```python
from build123d import *

# Parameters (mm, degrees)
SKETCH1_W           = 50.8
SKETCH1_H           = 50.8
SKETCH1_W_2         = 45.72
SKETCH1_H_2         = 45.72
BOSS_EXTRUDE1_DEPTH = 355.6
SKETCH2_R           = 14.2875
CUT_EXTRUDE1_DEPTH  = 50.8


with BuildPart() as part:
    # Sketch1 → Boss-Extrude1 (new body)
    with BuildSketch(Plane(origin=(0, 0, 0), x_dir=(1, 0, 0), z_dir=(0, 1, 0))):
        with Locations((25.4, -25.4)):
            Rectangle(SKETCH1_W, SKETCH1_H)
        with Locations((25.4, -25.4)):
            Rectangle(SKETCH1_W_2, SKETCH1_H_2, mode=Mode.SUBTRACT)
    extrude(amount=BOSS_EXTRUDE1_DEPTH)

    # Sketch2 → Cut-Extrude1 (cut)
    with BuildSketch(Plane.ZY):
        with Locations((25.4, 25.4)):
            Circle(SKETCH2_R)
    extrude(amount=-CUT_EXTRUDE1_DEPTH, mode=Mode.SUBTRACT)


solid = part.part
```
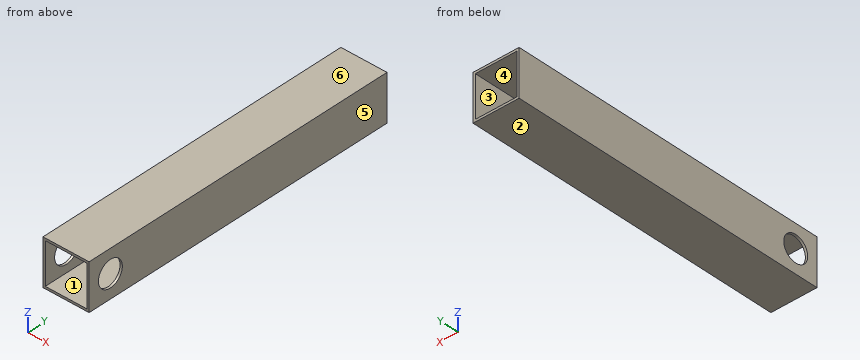
Verification items for the finished model (mm, model axes). Face numbers are marked on the shaded views. A direction names the side the tool comes from. Coordinates: 2 decimals unless noted, no trailing zeros. Write each loop counter-clockwise with the first axis right and the second up, starting at its lowest first coordinate (ties: lowest second). Pieces come first, ordered by that corner, then holes. Notation, with made-up numbers: M 22.25,-21 L 39.25,-21 A16 ccw 39.25,-15 Z; hole C 46,-20.75 d3. An arc over 180 degrees is marked long. Answer as a JSON object with one key per item and string values. Group by question number.
(1) Tool access check on the marked faces 1 and 2. Record the directions out of +Z, -Z, +X, -X, +Y, -Y that give a thin tool (end or side, any length) a straight path to the whole face; none if there is none.
(2) Material ranges on line 1 (X direction, y = 223, z = 12.5); line 2 (Y direction, x = 1.25, z = 25.4), recorded low to high.
(3) Cross-section at C-C, the plane y = 25.4. Record the cut outline in (x, z), and give its area (3 significant figures).
(4) Cross-section at A-A, the plane x = 24. Record the cut outline in (y, z), and give its area (3 significant figures).
(5) Cross-section at B-B, the plane z = 25.4. Record the cut outline in (x, y), and give its area (3 significant figures).
(6) Release check for a two-part mould opening along Z. For the marked faces 3, 4, 5 and 6 record: +Z half, -Z half, draft (parallel to the pull), parting line (faces both ways), or undercut.
(7) Cross-section at D-D, the plane z = 45. Record the cut outline in (x, y), and give its area (3 significant figures).
Reply:
{
 "1": {"face 1": "+Y, -Y", "face 2": "-Z, +X, -X, +Y, -Y"},
 "2": {"line 1": "0 to 2.54, 48.26 to 50.8", "line 2": "0 to 11.11, 39.69 to 355.6"},
 "3": {"outline": "M 0,0 L 50.8,0 L 50.8,11.11 L 48.26,11.11 L 48.26,2.54 L 2.54,2.54 L 2.54,11.11 L 0,11.11 Z; M 0,39.69 L 2.54,39.69 L 2.54,48.26 L 48.26,48.26 L 48.26,39.69 L 50.8,39.69 L 50.8,50.8 L 0,50.8 Z", "area": "345 mm²"},
 "4": {"outline": "M 0,0 L 355.6,0 L 355.6,2.54 L 0,2.54 Z; M 0,48.26 L 355.6,48.26 L 355.6,50.8 L 0,50.8 Z", "area": "1,810 mm²"},
 "5": {"outline": "M 0,0 L 2.54,0 L 2.54,11.11 L 0,11.11 Z; M 0,39.69 L 2.54,39.69 L 2.54,355.6 L 0,355.6 Z; M 48.26,0 L 50.8,0 L 50.8,11.11 L 48.26,11.11 Z; M 48.26,39.69 L 50.8,39.69 L 50.8,355.6 L 48.26,355.6 Z", "area": "1,660 mm²"},
 "6": {"face 3": "undercut", "face 4": "undercut", "face 5": "draft", "face 6": "+Z half"},
 "7": {"outline": "M 0,0 L 2.54,0 L 2.54,355.6 L 0,355.6 Z; M 48.26,0 L 50.8,0 L 50.8,355.6 L 48.26,355.6 Z", "area": "1,810 mm²"}
}
